from build123d import *

# Parameters (mm, degrees)
SKETCH1_W               = 50
SKETCH1_H               = 25
BOSS_EXTRUDE1_DEPTH     = 1200
SHELL1_T                = -2.5
CUT_EXTRUDE1_DEPTH      = 1201.419015069
CUT_EXTRUDE1_DEPTH_BACK = 1201.419015069
SKETCH2_R               = 7.5
SKETCH3_R               = 15.00115
CUT_EXTRUDE2_DEPTH      = 1201.593177499


with BuildPart() as part:
    # Sketch1 → Boss-Extrude1 (new body)
    with BuildSketch(Plane.XY):
        with Locations((3.266196349, 1.88172043)):
            Rectangle(SKETCH1_W, SKETCH1_H)
    extrude(amount=BOSS_EXTRUDE1_DEPTH)

    # Shell1
    shell1_openings = [part.faces().sort_by_distance(p)[0] for p in [
        (3.266196349, 1.88172043, 1200),
        (3.266196349, 1.88172043, 0),
    ]]
    offset(amount=SHELL1_T, openings=shell1_openings, kind=Kind.INTERSECTION)

    # Sketch2 → Cut-Extrude1 (cut, two sides: drawn at the far end of the back side and taken through both)
    with BuildSketch(Plane(origin=(0, 0, 0), x_dir=(1, 0, 0), z_dir=(0, 1, 0)).offset(-CUT_EXTRUDE1_DEPTH_BACK)):
        with Locations(Location((5.766196349, -900, 0), (0, 0, 90))):
            Circle(SKETCH2_R)
    extrude(amount=CUT_EXTRUDE1_DEPTH + CUT_EXTRUDE1_DEPTH_BACK, mode=Mode.SUBTRACT)

    # Sketch3 → Cut-Extrude2 (cut, through all)
    with BuildSketch(Plane(origin=(0, 14.38172043, 0), x_dir=(1, 0, 0), z_dir=(0, 1, 0))):
        with Locations(Location((3.266196349, -50, 0), (0, 0, 270))):
            Circle(SKETCH3_R)
        with Locations(Location((3.266196349, -1150, 0), (0, 0, 270))):
            Circle(SKETCH3_R)
    extrude(amount=-CUT_EXTRUDE2_DEPTH, mode=Mode.SUBTRACT)


solid = part.part
Source: CAD feature listing. Evaluate the final solid. Frame: model axes, mm. A direction names the side the tool comes from. Round coordinates to 2 decimals unless told otherwise and drop trailing zeros. Write each loop counter-clockwise with the first axis right and the second up, starting at its lowest first coordinate (ties: lowest second). Pieces come first, ordered by that corner, then holes. Notation, with made-up numbers: M 77,3 L 119,3 A7 ccw 119,15 Z; hole C -38,71.5 d11. An arc over 180 degrees is marked long. One line per item, written item: value. Start each with the question number.
Item 1: Ray query, L1, parallel to Y at x = -1.5, z = 484; L2, parallel to X at y = -4.75, z = 1001; L3, parallel to X at y = -10, z = 900. Return the intervals inside material, ascending. Write a range as from..to.
Item 2: Set-up query: faces 5 (the cylindrical face through (-2.479, -9.351, 63.857)), 6 (the flat face through (3, 11.882, 592)). Return all of +Z, -Z, +X, -X, +Y, -Y with unobstructed straight access to the full face (end or side cutting, diameter ignored); none if empty.
Item 3: Mould query, pull axis Z, two halves, no side actions, for faces 1 (the cylindrical face through (3.926, -9.351, 1135.013)), 2 (the flat face through (-21.734, 2, 592)), 3 (the cylindrical face through (3.926, 13.149, 1135.013)), 4 (the flat face through (3.1, 12.1, 1200)). Classes: pulls with the +Z half, pulls with the -Z half, needs draft (parallel to the pull), parting line crosses it, or undercut.
Item 4: Section query C-C (z = 762.5). Return the cut outline in (x, y).
Item 5: Section query B-B (z = 1150). Return the cut outline in (x, y).
Item 6: Section query A-A (y = 5.75). Return the cut outline in (x, z).
Result set:
1. L1: y = -10.62..-8.12, 11.88..14.38
1. L2: x = -21.73..-19.23, 25.77..28.27
1. L3: x = -21.73..-1.73, 13.27..28.27
2. face 5: +Y, -Y
2. face 6: +Z, -Z
3. face 1: undercut
3. face 2: needs draft
3. face 3: undercut
3. face 4: pulls with the +Z half
4. outline: M -21.73,-10.62 L 28.27,-10.62 L 28.27,14.38 L -21.73,14.38 Z; hole M -19.23,-8.12 L 25.77,-8.12 L 25.77,11.88 L -19.23,11.88 Z
5. outline: M -21.73,-10.62 L -11.73,-10.62 L -11.73,-8.12 L -19.23,-8.12 L -19.23,11.88 L -11.73,11.88 L -11.73,14.38 L -21.73,14.38 Z; M 18.27,-10.62 L 28.27,-10.62 L 28.27,14.38 L 18.27,14.38 L 18.27,11.88 L 25.77,11.88 L 25.77,-8.12 L 18.27,-8.12 Z
6. outline: M -21.73,0 L -19.23,0 L -19.23,1200 L -21.73,1200 Z; M 25.77,0 L 28.27,0 L 28.27,1200 L 25.77,1200 Z
